Check sheet for the drawn part. Datum: minimum x, y, z corner. Units: mm. A direction names the side the tool comes from. Round coordinates to 2 decimals unless told otherwise and drop trailing zeros. Order: outer loops, then holes, each group sorted by start corner. A loop starts at its lowest first (then second) coordinate and runs counter-clockwise, first axis right, second up. Notation, with made-up numbers: (-24.5, -22.5) -> (11.5, -22.5) arc R28 cw to (11.5, 5.5) -> close; hole circle Ø11 at (11, 51). An arc over 180 degrees is marked (long way). Answer as CSV lines item,"result". Start each with the question number.
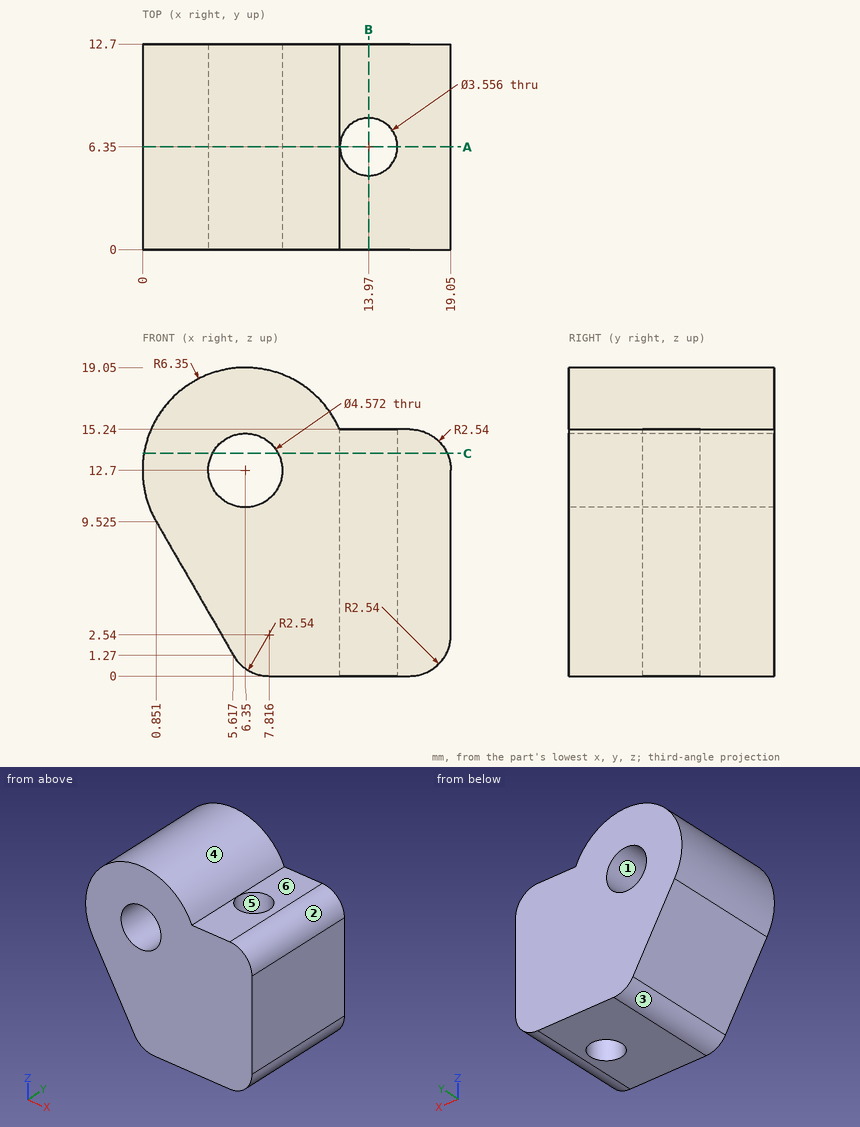
1) Section check B-B on x = 13.97. Record the cut outline in (y, z).
2) Mould release check, pull along X, two halves, no side actions. Record for the marked faces 1, 2, 3 and 4: released by +X, released by -X, zero draft, split by the parting line, or undercut.
3) Access from +Z, -Z, +X, -X, +Y, -Y to the whole of each face (thin tool, end or side, straight path). Record for the marked faces 5 and 6.
4) Section check A-A on y = 6.35. Count the separate pieces of the cut face and the enclosed holes in it, then the cut area to 3 significant figures.
5) Section check C-C on z = 13.75. Record the cut outline in (x, y).
6) Material ranges on line 1 along X through (y, z) = (10, 12.7); line 2 along Y through (x, z) = (13.97, 9.75); line 3 along Z through (x, y) = (15.5, 1.75), recorded low to high.
7) Depth check by flat-ended pin: pin 1 Ø3 at (x, y) = (13.97, 6.35) entering from +Z; pin 2 Ø3 at (y, z) = (9, 2.5) entering from -X; pin 3 Ø2 at (y, z) = (5, 15.5) entering from +X; pin 4 Ø3.5 at (x, y) = (14.5, 7) entering from +Z. Enter the tip coordinate at first touch or a pass-through.
Solutions:
1,outline,"(0, 0) -> (4.57, 0) -> (4.57, 15.24) -> (0, 15.24) -> close; (8.13, 0) -> (12.7, 0) -> (12.7, 15.24) -> (8.13, 15.24) -> close"
2,face 1,"undercut"
2,face 2,"released by +X"
2,face 3,"released by -X"
2,face 4,"split by the parting line"
3,face 5,"+Z, -Z"
3,face 6,"+Z, +X, +Y, -Y"
4,separate pieces,"2"
4,enclosed holes,"1"
4,area,"213 mm^2"
5,outline,"(0.09, 0) -> (4.32, 0) -> (4.32, 12.7) -> (0.09, 12.7) -> close; (8.38, 0) -> (18.82, 0) -> (18.82, 12.7) -> (8.38, 12.7) -> close; hole circle Ø3.56 at (13.97, 6.35)"
6,line 1,"x = 0 to 4.06, 8.64 to 19.05"
6,line 2,"y = 0 to 4.57, 8.13 to 12.7"
6,line 3,"z = 0 to 15.24"
7,pin 1,"passes through"
7,pin 2,"stops at x = 4.04"
7,pin 3,"stops at x = 18.3"
7,pin 4,"stops at z = 15.24"
